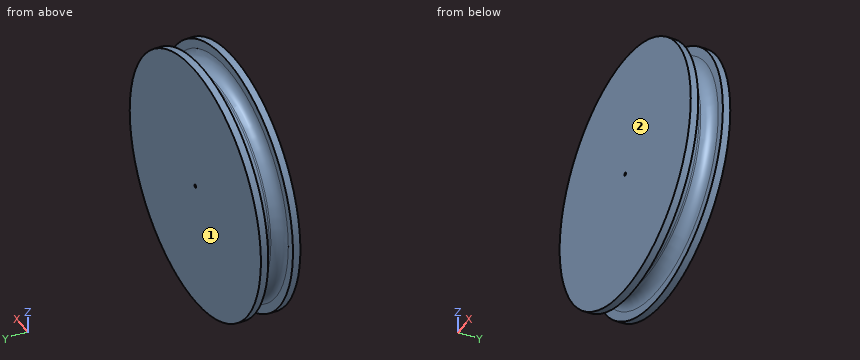
```python
from build123d import *

# Parameters (mm, degrees)
F0_R     = 38.75
F1_DEPTH = 6
F5_R     = 0.5
F6_DEPTH = 12.001


with BuildPart() as f1:
    # F0 (on Front) → F1 (new body, symmetric)
    with BuildSketch(Plane.XZ):
        Circle(F0_R)
    extrude(amount=F1_DEPTH, both=True)

    # F2 (on Right) → F4 (revolve, cut)
    with BuildSketch(Plane.YZ):
        with BuildLine():
            Line((3.75, 36), (3.75, 40))
            Line((3.75, 40), (-3.75, 40))
            Line((-3.75, 40), (-3.75, 36))
            ThreePointArc((-3.75, 36), (-2.724874, 33.525126), (-0.25, 32.5))
            Line((-0.25, 32.5), (0.25, 32.5))
            ThreePointArc((0.25, 32.5), (2.724874, 33.525126), (3.75, 36))
        make_face()
    revolve(axis=Axis((0, -2.011297, 0), (0, -1, 0)), mode=Mode.SUBTRACT)

    # F5 (on face) → F6 (cut, through all)
    with BuildSketch(Plane(origin=(0, 6, 0), x_dir=(-1, 0, 0), z_dir=(0, 1, 0))):
        Circle(F5_R)
    extrude(amount=-F6_DEPTH, mode=Mode.SUBTRACT)


solid = f1.part
```
Geometry: final body of the model. Coordinates: model frame, mm. Face numbers are marked on the shaded views. Round coordinates to 2 decimals unless told otherwise and drop trailing zeros. Write each loop counter-clockwise with the first axis right and the second up, starting at its lowest first coordinate (ties: lowest second). Pieces come first, ordered by that corner, then holes.
Item 1: Material intervals for L1, parallel to Y at x = 32.5, z = 6; L2, parallel to Y at x = 16, z = -34; L3, parallel to Z at x = 0, y = -3.25, sorted ascending.
Item 2: Pin query (flat end, axial travel): P1, Ø6, axis at x = -22.5, y = 1.5, coming from the +Z side; P2, Ø1.5, axis at y = 0, z = 30, coming from the +X side; P3, Ø5, axis at x = -12, y = 4.5, coming from the -Z side. Return the tip coordinate at first contact, or that it passes through.
Item 3: Mould query, pull axis Y, two halves, no side actions, for the marked faces 1 and 2. Classes: +Y half, -Y half, draft (parallel to the pull), parting line (faces both ways), or undercut.
Item 4: Section query A-A (y = -5). Return loops of the section in (x, z).
Completed:
1. L1: y = -6 to -2.13, 2.13 to 6
1. L2: y = -6 to -3.75, 3.75 to 6
1. L3: z = -34.2 to -0.5, 0.5 to 34.2
2. P1: stops at z = 32.87
2. P2: stops at x = 14.17
2. P3: stops at z = -37.57
3. face 1: +Y half
3. face 2: -Y half
4. outline: circle Ø77.5 at (0, 0); hole circle Ø1 at (0, 0)
